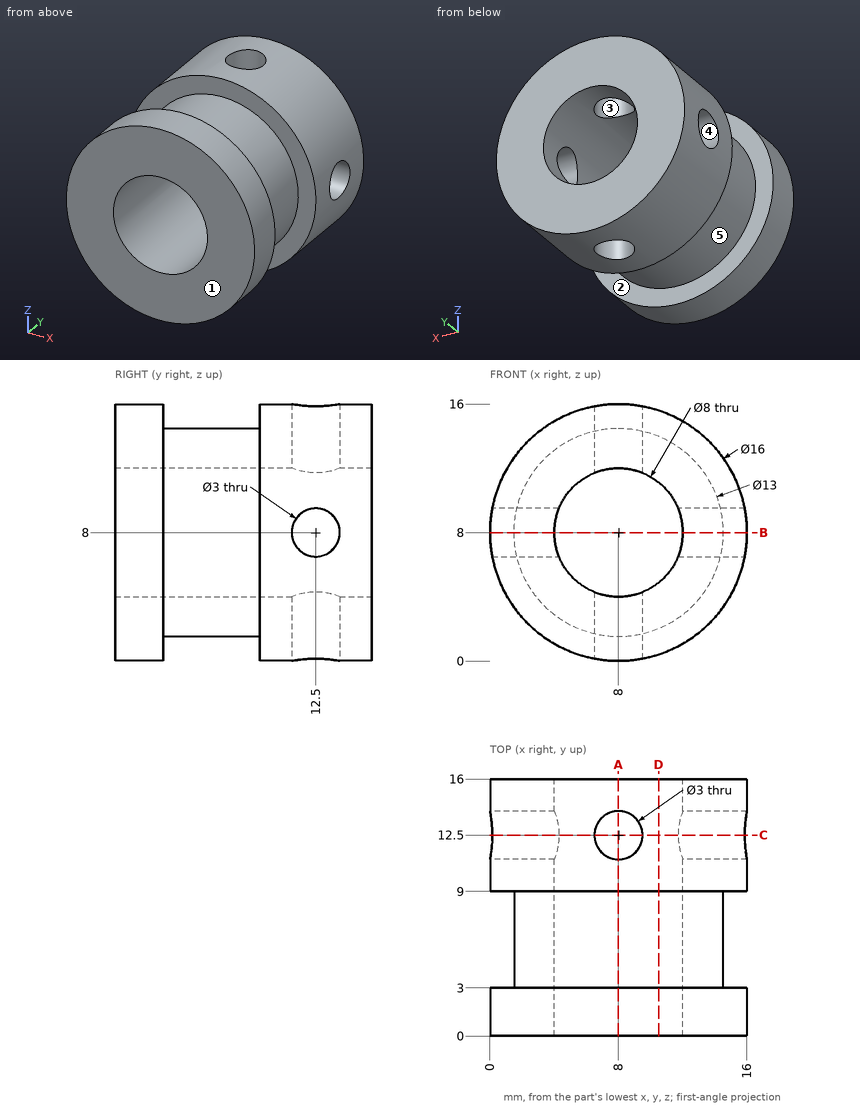
The figure shows three views and two pictorial views of one solid part (mm, origin at its lowest corner). Answer the questions. A direction names the side the tool comes from. Round coordinates to 2 decimals unless told otherwise and drop trailing zeros. Order: outer loops, then holes, each group sorted by start corner. A loop starts at its lowest first (then second) coordinate and runs counter-clockwise, first axis right, second up. Notation, with made-up numbers: M 61,-30 L 98,-30 A18 cw 98,-15 Z; hole C 87,49.25 d8. An arc over 180 degrees is marked long. Put each result on its own line as item: value. Start each with the question number.
Q1. A tool of negligible diameter and unlimited length cuts with its end or side. For the marked faces 1 and 2, from which of +Z, -Z, +X, -X, +Y, -Y can it reach the whole face along a straight path? Write none if from no direction.
Q2. Flat-ended cylindrical pins translate along their axes: pin 1 (5 mm diameter, centred on x = 9.5, z = 6.5, fed in from +Y); pin 2 (1 mm diameter, centred on y = 11.5, z = 14.5, fed in from +X); pin 3 (4 mm diameter, centred on x = 10.5, y = 9, fed in from +Z); pin 4 (1.5 mm diameter, centred on x = 10, y = 11.5, fed in from -Z). Find the tip coordinate at first contact, or state that the pin passes through.
Q3. Section B-B, the plane z = 8 is taken. Write down the section's boundary in (x, y), and give its area (3 significant figures).
Q4. For a pull along X with two mould halves and no side action, classify the marked faces 3, 4 and 5 as pulls with the +X half, pulls with the -X half, needs draft (parallel to the pull), parting line crosses it, or undercut.
Q5. Section A-A, the plane x = 8 is taken. Write down the section's boundary in (y, z).
Q6. Section D-D, the plane x = 10.5 is taken. Write down the section's boundary in (y, z).
Q7. Straight lines are drawn through the part: L1, parallel to Y at x = 6, z = 14.75; L2, parallel to Y at x = 7.75, z = 15.75; L3, parallel to X at y = 5, z = 8. For each, find the intervals that lie inside material, in ascending order. Write a range as [from, to].
Q8. Section C-C, the plane y = 12.5 is taken. Write down the section's boundary in (x, z).
Findings below:
1. face 1: +Z, -Z, +X, -X, -Y
1. face 2: none
2. pin 1: stops at y = 16
2. pin 2: stops at x = 13.29
2. pin 3: stops at z = 15.98
2. pin 4: stops at z = 0.1
3. outline: M 0,0 L 4,0 L 4,11 L 0,11 L 0,9 L 1.5,9 L 1.5,3 L 0,3 Z; M 0,14 L 4,14 L 4,16 L 0,16 Z; M 12,0 L 16,0 L 16,3 L 14.5,3 L 14.5,9 L 16,9 L 16,11 L 12,11 Z; M 12,14 L 16,14 L 16,16 L 12,16 Z
3. area: 86.0 mm^2
4. face 3: undercut
4. face 4: needs draft
4. face 5: parting line crosses it
5. outline: M 0,0 L 3,0 L 3,1.5 L 9,1.5 L 9,0 L 11,0 L 11,4 L 0,4 Z; M 0,12 L 11,12 L 11,16 L 9,16 L 9,14.5 L 3,14.5 L 3,16 L 0,16 Z; M 14,0 L 16,0 L 16,4 L 14,4 Z; M 14,12 L 16,12 L 16,16 L 14,16 Z
6. outline: M 0,0.4 L 3,0.4 L 3,2 L 9,2 L 9,0.4 L 16,0.4 L 16,4.88 L 0,4.88 Z; M 0,11.12 L 16,11.12 L 16,15.6 L 9,15.6 L 9,14 L 3,14 L 3,15.6 L 0,15.6 Z
7. L1: y = [0, 3], [9, 16]
7. L2: y = [0, 3], [9, 11.02], [13.98, 16]
7. L3: x = [1.5, 4], [12, 14.5]
8. outline: M 0.14,6.5 A8 ccw 6.5,0.14 L 6.5,4.29 A4 cw 4.29,6.5 Z; M 0.14,9.5 L 4.29,9.5 A4 cw 6.5,11.71 L 6.5,15.86 A8 ccw Z; M 9.5,0.14 A8 ccw 15.86,6.5 L 11.71,6.5 A4 cw 9.5,4.29 Z; M 9.5,11.71 A4 cw 11.71,9.5 L 15.86,9.5 A8 ccw 9.5,15.86 Z
